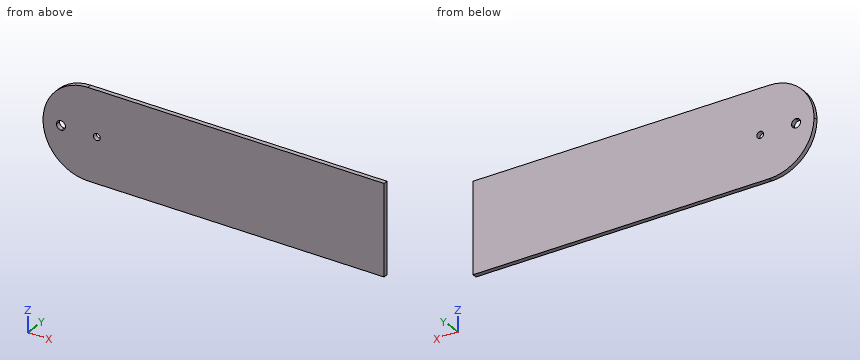
```python
from build123d import *

# Parameters (mm, degrees)
F1_DEPTH = 3.175


# Not quite as in the source:
# - a feature names something its author has since deleted; it is built from what else it names


with BuildPart() as f1:
    # F0 (on Front) → F1 (new body)
    with BuildSketch(Plane.XZ):
        with BuildLine():
            ThreePointArc((0, 31.75), (9.2993596973, 9.2993596973), (31.75, 0))
            Line((31.75, 0), (241.3, 0))
            Line((241.3, 0), (241.3, 63.5))
            Line((241.3, 63.5), (31.75, 63.5))
            ThreePointArc((31.75, 63.5), (9.2993596973, 54.2006403027), (0, 31.75))
        make_face()
        with BuildLine():
            ThreePointArc((12.8984375, 28.5812072396), (10.5262260999, 29.4358409667), (9.525, 31.75))
            ThreePointArc((9.525, 31.75), (10.5262260999, 34.0641590333), (12.8984375, 34.9187927604))
            ThreePointArc((12.8984375, 34.9187927604), (39.6875, 57.1003420835), (63.5, 31.75))
            ThreePointArc((63.5, 31.75), (39.6875, 6.3996579165), (12.8984375, 28.5812072396))
        make_face(mode=Mode.SUBTRACT)
        with BuildLine():
            ThreePointArc((63.5, 31.75), (39.6875, 57.1003420835), (12.8984375, 34.9187927604))
            ThreePointArc((12.8984375, 34.9187927604), (15.0141590333, 33.9237739001), (15.875, 31.75))
            ThreePointArc((15.875, 31.75), (15.0141590333, 29.5762260999), (12.8984375, 28.5812072396))
            ThreePointArc((12.8984375, 28.5812072396), (39.6875, 6.3996579165), (63.5, 31.75))
        make_face()
        with BuildLine():
            ThreePointArc((40.48125, 31.75), (38.1, 29.36875), (35.71875, 31.75))
            ThreePointArc((35.71875, 31.75), (38.1, 34.13125), (40.48125, 31.75))
        make_face(mode=Mode.SUBTRACT)
    extrude(amount=F1_DEPTH)


solid = f1.part
```
Source: CAD feature listing. Evaluate the final solid. Frame: model axes, mm. Give positions to 0.01 mm unless a question says otherwise; leave off trailing zeros. Write each loop counter-clockwise with the first axis right and the second up, starting at its lowest first coordinate (ties: lowest second). Pieces come first, ordered by that corner, then holes.
1. Section query B-B (y = -2.05). Count the separate pieces of the cut face and the enclosed holes in it, then the cut area to 3 significant figures.
2. Material intervals for line 1 along X through (y, z) = (-2.1, 31.75) (3 decimals); line 2 along Z through (x, y) = (38.1, -0.85); line 3 along X through (y, z) = (-1.7, 51), sorted ascending.
3. Section query D-D (z = 57). Return the cut outline in (x, y) (3 decimals), then the cut area to 3 significant figures.
4. Section query C-C (z = 9). Return the cut outline in (x, y) (3 decimals).
5. First-contact query: pin 1 (4 mm diameter, centred on x = 38.1, z = 31.75, fed in from -Y). Flat tip, straight axial feed; report the tip coordinate or a pass-through.
6. Section query A-A (x = 38.1). Return the cut outline in (y, z) (3 decimals), then the cut area to 3 significant figures.
Output values:
1. separate pieces: 1
1. enclosed holes: 2
1. area: 14,800 mm2
2. line 1: x = 0 to 9.525, 15.875 to 35.719, 40.481 to 241.3
2. line 2: z = 0 to 29.37, 34.13 to 63.5
2. line 3: x = 6.5 to 241.3
3. outline: (12.502, -3.175) - (241.3, -3.175) - (241.3, 0) - (12.502, 0) - close
3. area: 726 mm2
4. outline: (9.603, -3.175) - (241.3, -3.175) - (241.3, 0) - (9.603, 0) - close
5. pin 1: passes through
6. outline: (-3.175, 0) - (0, 0) - (0, 29.369) - (-3.175, 29.369) - close; (-3.175, 34.131) - (0, 34.131) - (0, 63.5) - (-3.175, 63.5) - close
6. area: 186 mm2
